The model under review builds one solid part; all positions refer to its coordinate system, in mm. A direction names the side the tool comes from. Round coordinates to 2 decimals unless told otherwise and drop trailing zeros. Order: outer loops, then holes, each group sorted by start corner. A loop starts at its lowest first (then second) coordinate and runs counter-clockwise, first axis right, second up.
Autodesk Inventor part; units mm, degrees
ref_plane "YZ Plane" through (0, 0, 0) normal (1, 0, 0) x (0, 1, 0)
ref_plane "XZ Plane" through (0, 0, 0) normal (0, 1, 0) x (-1, 0, 0)
ref_plane "XY Plane" through (0, 0, 0) normal (0, 0, 1) x (1, 0, 0)
sketch "Sketch1" plane through (0, 0, 0) normal (0, 0, 1) x (1, 0, 0)
  arc A0 (-2.4, -4.5) -> (-2.4, 4.5) centre (0, 0) ccw
  line L0 (-2.4, 4.5) -> (-12, 4.5)
  line L1 (-12, 4.5) -> (-12, 9)
  line L2 (-12, 9) -> (5, 9)
  line L3 (5, -9) -> (-12, -9)
  line L4 (-12, -9) -> (-12, -4.5)
  line L5 (-12, -4.5) -> (-2.4, -4.5)
  line L6 (5, 9) -> (5, 13.25)
  line L7 (5, -9) -> (5, -13.25)
  line L8 (5, 13.25) -> (9, 13.25)
  line L9 (9, 13.25) -> (9, -13.25)
  line L10 (9, -13.25) -> (5, -13.25)
  dimension "d0" = 10.2
  dimension "d1" = 9
  dimension "d2" = 12
  dimension "d3" = 9
  dimension "d7" = 26.5
  dimension "d8" = 4.25
  dimension "d9" = 4
  dimension "d10" = 5
extrude "Extrusion1" add sketch "Sketch1" along normal blind 10
sketch "Sketch4" plane through (5, 13.25, 0) normal (0, 1, 0) x (1, 0, 0)
  line L0 (4, 0) -> (4, -10)
  line L1 (4, 0) -> (4, -10)
  line L2 (18, -3) -> (18, -7)
  line L3 (18, -7) -> (4, -7)
  line L4 (18, -3) -> (4, -3)
  line L5 (4, 0) -> (0, 0)
  point P0 (-5, 0)
  dimension "d24" = 4
  dimension "d47" = 14
  dimension "d48" = 3
extrude "Extrusion4" add sketch "Sketch4" against normal up to surface (26.5 mm away)
sketch "Sketch5" plane through (9, 13.25, 7) normal (0, 0, 1) x (1, 0, 0)
  line L0 (0, -26.5) -> (14, -26.5)
  line L1 (14, 0) -> (14, -26.5)
  line L2 (0, 0) -> (14, 0)
  circle A0 centre (9, -3.75) radius 1.75
  circle A1 centre (9, -22.75) radius 1.75
  point P0 (-9, -13.25)
  dimension "d27" = 3.5
  dimension "d28" = 3.75
  dimension "d29" = 3.75
  dimension "d30" = 5
extrude "Extrusion5" cut sketch "Sketch5" against normal up to next
sketch "Sketch6" plane through (-12, -9, 0) normal (0, -1, 0) x (1, 0, 0)
  line L0 (0, 10) -> (17, 10)
  line L1 (0, 0) -> (0, 10)
  circle A0 centre (3, 5) radius 1.75
  point P0 (12, 0)
  dimension "d33" = 3.5
  dimension "d34" = 3
  dimension "d35" = 5
extrude "Extrusion6" cut sketch "Sketch6" against normal up to surface (18 mm away)
sketch "Sketch7" plane through (-12, 9, 0) normal (0, 1, 0) x (1, 0, 0)
  circle A0 centre (3, -5) radius 1.75
  line L0 (3, -8.3486) -> (0.1, -6.6743)
  line L1 (0.1, -6.6743) -> (0.1, -3.3257)
  line L2 (0.1, -3.3257) -> (3, -1.6514)
  line L3 (3, -1.6514) -> (5.9, -3.3257)
  line L4 (5.9, -3.3257) -> (5.9, -6.6743)
  line L5 (5.9, -6.6743) -> (3, -8.3486)
  point P0 (12, 0)
  dimension "d38" = 5.8
extrude "Extrusion7" cut sketch "Sketch7" against normal blind 2.5
sketch "Sketch8" plane through (9, 13.25, 7) normal (0, 0, 1) x (1, 0, 0)
  circle A0 centre (9, -3.75) radius 1.75
  circle A1 centre (9, -22.75) radius 1.75
  line L0 (5.6514, -22.75) -> (7.3257, -19.85)
  line L1 (7.3257, -19.85) -> (10.6743, -19.85)
  line L2 (10.6743, -19.85) -> (12.3486, -22.75)
  line L3 (12.3486, -22.75) -> (10.6743, -25.65)
  line L4 (10.6743, -25.65) -> (7.3257, -25.65)
  line L5 (7.3257, -25.65) -> (5.6514, -22.75)
  line L6 (5.6514, -3.75) -> (7.3257, -0.85)
  line L7 (7.3257, -0.85) -> (10.6743, -0.85)
  line L8 (10.6743, -0.85) -> (12.3486, -3.75)
  line L9 (12.3486, -3.75) -> (10.6743, -6.65)
  line L10 (10.6743, -6.65) -> (7.3257, -6.65)
  line L11 (7.3257, -6.65) -> (5.6514, -3.75)
  point P0 (-9, -13.25)
  dimension "d41" = 5.8
extrude "Extrusion8" cut sketch "Sketch8" against normal blind 2.5
chamfer "Chamfer1" distance 2 angle 45 2 edges at (9, 0, 7) (9, 0, 3)
properties part number "ZAxisEndstopMount"
(1) Consider section B-B (y = 7.25). Write out the cut boundary in (x, z), and give its area (3 significant figures).
Data:
outline: (-12, 0) - (9, 0) - (9, 1) - (11, 3) - (23, 3) - (23, 7) - (20.05, 7) - (20.05, 4.5) - (15.95, 4.5) - (15.95, 7) - (11, 7) - (9, 9) - (9, 10) - (-12, 10) - close; hole (-11.9, 3.33) - (-9, 1.65) - (-6.1, 3.33) - (-6.1, 6.67) - (-9, 8.35) - (-11.9, 6.67) - close
area: 231 mm2
(2) Consider section C-C (y = -2.5). Write out the cut boundary in (x, z), and give its area (3 significant figures).
Data:
outline: (4.45, 0) - (9, 0) - (9, 1) - (11, 3) - (23, 3) - (23, 7) - (11, 7) - (9, 9) - (9, 10) - (4.45, 10) - close
area: 106 mm2
(3) Insertion check: pin 1 (13 mm diameter, centred on x = 18, y = 0, fed in from -Z); pin 2 (3 mm diameter, centred on x = -7.5, z = 3.5, fed in from -Y); pin 3 (9.5 mm diameter, centred on x = 19.5, y = 0.5, fed in from +Z). Each pin has a flat end and moves straight along its axis. Give the tip position at first contact, or say it passes through.
Data:
pin 1: stops at z = 3
pin 2: stops at y = -9
pin 3: stops at z = 7
(4) Draft analysis for pull direction X (two halves, no side actions). For faces 6 (the flat face through (-6.1, 8, 5)), 7 (the flat face through (15.477, -8.07, 5.768)), 8 (the flat face through (-12, -7, 5)), 9 (the flat face through (12, -13.25, 5)), state which applies: pulls with the +X half, pulls with the -X half, needs draft (parallel to the pull), parting line crosses it, or undercut.
Data:
face 6: undercut
face 7: undercut
face 8: pulls with the -X half
face 9: needs draft
(5) For faces 1 (the flat face through (18, 6.6, 6)), 2 (the flat face through (17, 0, 3)), 3 (the flat face through (-3, -9, 5)), 4 (the flat face through (5, 11, 5)), 5 (the cylindrical face through (-8.19, -6.78, 3.45)), list the 3-axis set-ups (+Z, -Z, +X, -X, +Y, -Y) from which the entire face can be reached by the end or side of a thin tool; tool diameter is ignored.
Data:
face 1: +Z
face 2: -Z, +X, +Y, -Y
face 3: +Z, -Z, -X, -Y
face 4: +Z, -Z, -X, +Y
face 5: +Y, -Y
(6) Consider section A-A (z = 3.75). Write out the cut boundary in (x, y), and give its area (3 significant figures).
Data:
outline: (-12, -9) - (-10.22, -9) - (-10.22, -4.5) - (-12, -4.5) - close; (-12, 4.5) - (-10.22, 4.5) - (-10.22, 6.5) - (-11.9, 6.5) - (-11.9, 9) - (-12, 9) - close; (-7.78, -9) - (5, -9) - (5, -13.25) - (23, -13.25) - (23, 13.25) - (5, 13.25) - (5, 9) - (-6.1, 9) - (-6.1, 6.5) - (-7.78, 6.5) - (-7.78, 4.5) - (-2.4, 4.5) arc R5.1 cw (long way) to (-2.4, -4.5) - (-7.78, -4.5) - close; hole circle Ø3.5 at (18, -9.5); hole circle Ø3.5 at (18, 9.5)
area: 583 mm2
(7) Consider section D-D (x = 15.5). Write out the cut boundary in (y, z), and give its area (3 significant figures).
Data:
outline: (-13.25, 3) - (13.25, 3) - (13.25, 7) - (10.97, 7) - (10.97, 4.5) - (8.03, 4.5) - (8.03, 7) - (-8.03, 7) - (-8.03, 4.5) - (-10.97, 4.5) - (-10.97, 7) - (-13.25, 7) - close
area: 91.3 mm2
(8) To check wall thickness, follow probe 1 along Y at (x, z) = (18, 3.9); probe 2 along Z at (x, y) = (-9, -5); probe 3 along X at (y, z) = (6.1, 5). State the ranges of each line that lie inside material, in increasing order.
Data:
probe 1: y = -13.25 to -11.25, -7.75 to 7.75, 11.25 to 13.25
probe 2: z = 0 to 3.25, 6.75 to 10
probe 3: x = -12 to -10.75, -7.25 to 23
